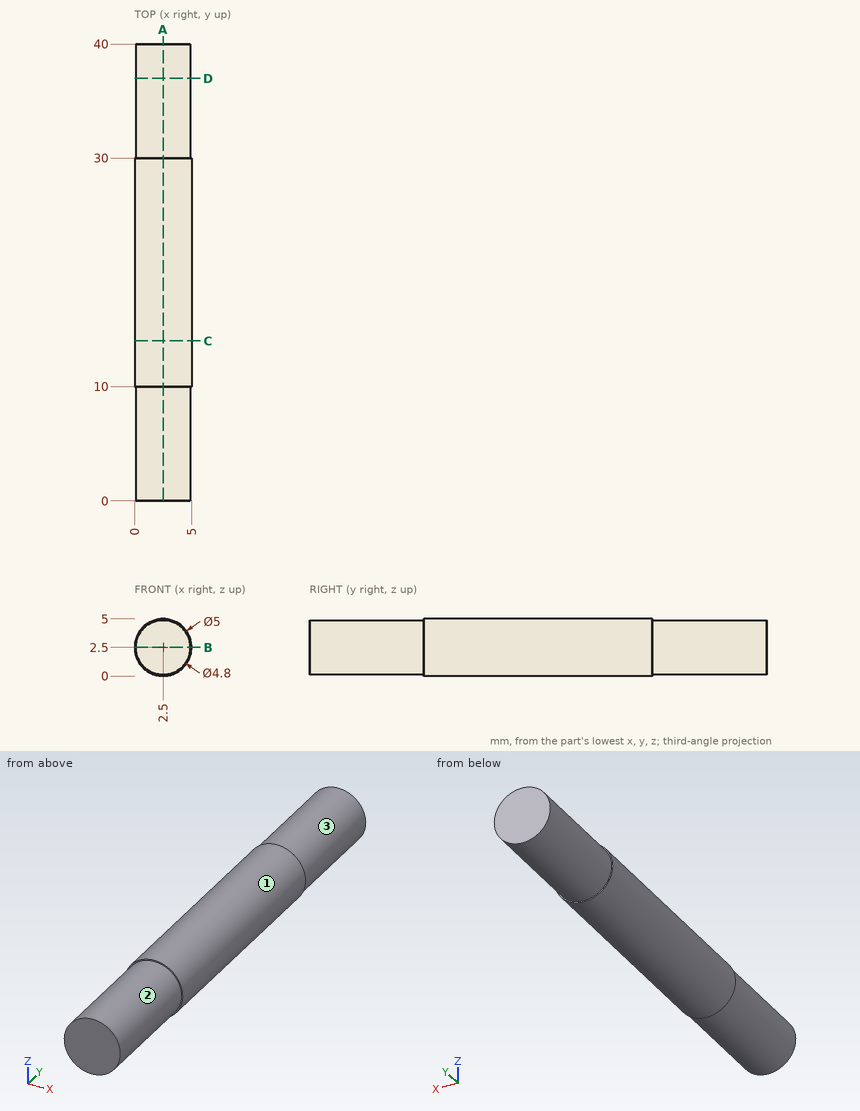
For this review, use the dimensioned drawing (mm, ordinates from the lowest corner) and the shaded views. A direction names the side the tool comes from. Give positions to 0.01 mm unless a question says otherwise; leave off trailing zeros. Order: outer loops, then holes, each group sorted by start corner. A loop starts at its lowest first (then second) coordinate and runs counter-clockwise, first axis right, second up. Notation, with made-up numbers: (63.25, -25) - (105.25, -25) arc R13 ccw to (105.25, -1) - close; hole circle Ø9 at (-0.75, 9). An arc over 180 degrees is marked (long way). Use CSV: the item, a comma, the result in double quotes. Start each with the question number.
Q1. Take a section at C-C (y = 14). State the section outline as (x, z) points.
Q2. Take a section at B-B (z = 2.5). State the section outline as (x, y) points, and give its area (3 significant figures).
Q3. Take a section at A-A (x = 2.5). State the section outline as (y, z) points, and give its area (3 significant figures).
Q4. For P1, Ø1, axis at y = 11.5, z = 3.5, coming from the -X side, flat-tipped, find the tip position at first contact; note if it passes through.
Q5. Take a section at D-D (y = 37). State the section outline as (x, z) points.
Q6. For line 1 (Z direction, x = 2.6, y = 21); line 2 (X direction, y = 23, z = 3.3); line 3 (X direction, y = 31, z = 0.6), list the stretches that pass through material, from the lowest coordinate up.
Q7. Machinability: for the marked faces 1, 2 and 3, which of the approach directions +Z, -Z, +X, -X, +Y, -Y give a long, thin tool a straight path to every point of the face, cutting with its end or side? Answer none if there is none.
Calculated:
1,outline,"circle Ø5 at (2.5, 2.5)"
2,outline,"(0, 10) - (0.1, 10) - (0.1, 0) - (4.9, 0) - (4.9, 10) - (5, 10) - (5, 30) - (4.9, 30) - (4.9, 40) - (0.1, 40) - (0.1, 30) - (0, 30) - close"
2,area,"196 mm²"
3,outline,"(0, 0.1) - (10, 0.1) - (10, 0) - (30, 0) - (30, 0.1) - (40, 0.1) - (40, 4.9) - (30, 4.9) - (30, 5) - (10, 5) - (10, 4.9) - (0, 4.9) - close"
3,area,"196 mm²"
4,P1,"stops at x = 0.05"
5,outline,"circle Ø4.8 at (2.5, 2.5)"
6,line 1,"z = 0 to 5"
6,line 2,"x = 0.13 to 4.87"
6,line 3,"x = 1.03 to 3.97"
7,face 1,"+Y, -Y"
7,face 2,"-Y"
7,face 3,"+Y"
